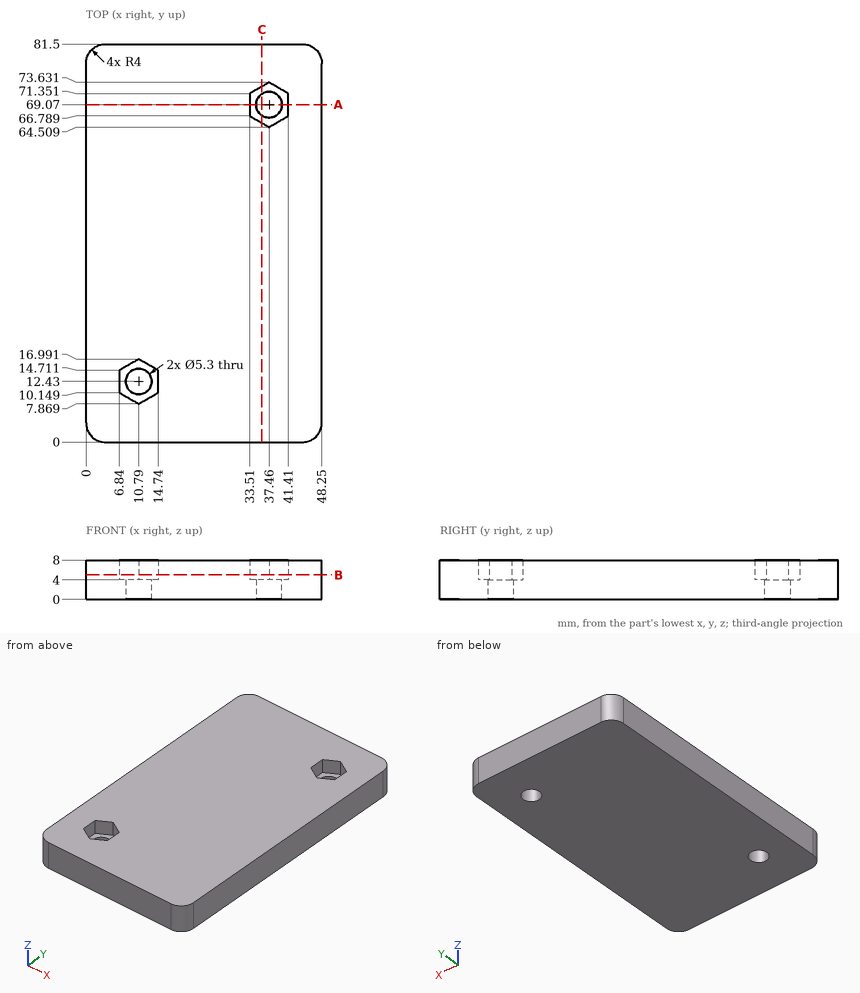
Answer from the drawing. Dimensions are ordinates in mm from the lowest x, y and z of the part. Coordinates: 2 decimals unless noted, no trailing zeros. Loops run counter-clockwise (first coordinate to the right, second up) from the corner with the lowest first, then second, coordinate; pieces in that order, holes last. Notation, with made-up numbers: (37, 70.25) - (87, 70.25) arc R13 cw to (87, 74.25) - close; hole circle Ø7 at (-20, -26). An arc over 180 degrees is marked (long way). Answer in a Markdown table with one row per item.
1. Find section B-B, the plane z = 5. Write down the section's boundary in (x, y), then the cut area to 3 significant figures.
Conclusion:
| item | result |
|---|---|
| outline | (0, 4) arc R4 ccw to (4, 0) - (44.25, 0) arc R4 ccw to (48.25, 4) - (48.25, 77.5) arc R4 ccw to (44.25, 81.5) - (4, 81.5) arc R4 ccw to (0, 77.5) - close; hole (6.84, 10.15) - (10.79, 7.87) - (14.74, 10.15) - (14.74, 14.71) - (10.79, 16.99) - (6.84, 14.71) - close; hole (33.51, 66.79) - (37.46, 64.51) - (41.41, 66.79) - (41.41, 71.35) - (37.46, 73.63) - (33.51, 71.35) - close |
| area | 3,810 mm² |
2. Straight lines are drawn through the part: line 1 (X direction, y = 69.07, z = 0.95); line 2 (Y direction, x = 37.46, z = 2.7); line 3 (X direction, y = 12.43, z = 2.8). For each, find the intervals that lie inside material, in ascending order.
Conclusion:
| item | result |
|---|---|
| line 1 | x = 0 to 34.81, 40.11 to 48.25 |
| line 2 | y = 0 to 66.42, 71.72 to 81.5 |
| line 3 | x = 0 to 8.14, 13.44 to 48.25 |
3. Find section A-A, the plane y = 69.07. Write down the section's boundary in (x, z).
Conclusion:
| item | result |
|---|---|
| outline | (0, 0) - (34.81, 0) - (34.81, 4) - (33.51, 4) - (33.51, 8) - (0, 8) - close; (40.11, 0) - (48.25, 0) - (48.25, 8) - (41.41, 8) - (41.41, 4) - (40.11, 4) - close |
4. Find section C-C, the plane x = 36. Write down the section's boundary in (y, z).
Conclusion:
| item | result |
|---|---|
| outline | (0, 0) - (66.86, 0) - (66.86, 4) - (65.35, 4) - (65.35, 8) - (0, 8) - close; (71.28, 0) - (81.5, 0) - (81.5, 8) - (72.79, 8) - (72.79, 4) - (71.28, 4) - close |
5. Given pin 1 (2.5 mm diameter, centred on x = 36, y = 68, fed in from +Z); pin 2 (4 mm diameter, centred on y = 67.5, z = 3, fed in from -X), each flat-ended and moving along its own axis, determine where each tip first touches the part or whether it passes through.
Conclusion:
| item | result |
|---|---|
| pin 1 | stops at z = 4 |
| pin 2 | stops at x = 0 |
